Autodesk Fusion 360 part; units mm, degrees
sketch "Sketch1" plane through (0, 0, 0) normal (0, 0, 1) x (1, 0, 0)
  line L0 (55, 35) -> (117.913, 35)
  line L1 (117.913, 35) -> (117.913, -30.294)
  line L2 (117.913, -30.294) -> (55, -30.294)
  line L3 (55, -30.294) -> (55, 35)
  line L4 (44.5, -40.794) -> (127.413, -40.794)
  line L5 (127.413, -40.794) -> (127.413, 44.5)
  line L6 (127.413, 44.5) -> (44.5, 44.5)
  line L7 (44.5, 44.5) -> (44.5, -40.794)
  circle A0 centre (49.5, -35.794) radius 1.7
  circle A1 centre (49.5, 39.5) radius 1.7
  circle A2 centre (122.413, 39.5) radius 1.7
  circle A3 centre (122.413, -35.794) radius 1.7
  circle A4 centre (49.5, -35.794) radius 3
  circle A5 centre (49.5, 39.5) radius 3
  circle A6 centre (122.413, 39.5) radius 3
  circle A7 centre (122.413, -35.794) radius 3
  dimension "d1" = 62.913
  dimension "d2" = 65.294
  dimension "d3" = 82.913
  dimension "d4" = 85.294
  dimension "d5" = 9.5
  dimension "d6" = 9.5
  dimension "d7" = 3.4
  dimension "d8" = 3.4
  dimension "d9" = 3.4
  dimension "d10" = 3.4
  dimension "d11" = 5
  dimension "d12" = 5
  dimension "d13" = 5
  dimension "d14" = 5
  dimension "d15" = 5
  dimension "d16" = 5
  dimension "d17" = 5
  dimension "d18" = 5
  dimension "d19" = 6
  dimension "d20" = 6
  dimension "d21" = 6
  dimension "d22" = 6
extrude "Extrude1" add sketch "Sketch1" along normal blind 9.9 from surface at 3.1 contours A4 | A5 | A6 | A7 makes body 1 at (123.2255, -32.9061, 9.7) makes body 2 at (123.2255, 42.3879, 9.7) makes body 3 at (46.5037, -35.9435, 9.7) makes body 4 at (46.5037, 39.3505, 9.7)
extrude "Extrude2" add sketch "Sketch1" along normal blind 13 contours L4 L5 L6 L7 bodies 1 2 3 4
extrude "Extrude3" add sketch "Sketch1" along normal blind 3 contours L0 L1 L2 L3 bodies 1
sketch "Sketch2" plane through (0, 0, 13) normal (0, 0, 1) x (-1, 0, 0)
  circle A0 centre (-122.413, 35.794) radius 1.7
  circle A1 centre (-49.5, -39.5) radius 1.7
  line L0 (-117.913, 30.294) -> (-55, 30.294)
  line L1 (-55, 30.294) -> (-55, -35)
  line L2 (-55, -35) -> (-117.913, -35)
  line L3 (-117.913, -35) -> (-117.913, 30.294)
  line L4 (-44.5, -44.5) -> (-44.5, 40.794)
  line L5 (-44.5, 40.794) -> (-127.413, 40.794)
  line L6 (-127.413, 40.794) -> (-127.413, -44.5)
  line L7 (-127.413, -44.5) -> (-44.5, -44.5)
  circle A2 centre (-122.413, -39.5) radius 1.7
  circle A3 centre (-49.5, 35.794) radius 1.7
  line L8 (-76.7065, -44.5) -> (-95.2065, -44.5)
  line L9 (-95.2065, -44.5) -> (-95.2065, -35)
  line L10 (-95.2065, -35) -> (-76.7065, -35)
  line L11 (-76.7065, -35) -> (-76.7065, -44.5)
  line L12 (-44.5, -44.5) -> (-44.5, 40.794)
  dimension "d30" = 18.5
  dimension "d31" = 32.2065
extrude "Extrude4" cut sketch "Sketch2" against normal blind 7.5 contours L2 L7 L8 L9 L10 L11 bodies 1
fillet "Fillet1" radius 5 4 edges at (44.5, 44.5, 6.5) (44.5, -40.794, 6.5) (127.413, 44.5, 6.5) (127.413, -40.794, 6.5) on bodies 1
sketch "Sketch3" plane through (0, 0, 13) normal (0, 0, 1) x (-1, 0, 0)
  circle A0 centre (-49.5, 35.794) radius 1.7
  circle A1 centre (-122.413, -39.5) radius 1.7
  arc A2 (-122.413, 40.794) -> (-127.413, 35.794) centre (-122.413, 35.794) ccw
  line L0 (-127.413, 35.794) -> (-127.413, -39.5)
  arc A3 (-127.413, -39.5) -> (-122.413, -44.5) centre (-122.413, -39.5) ccw
  line L1 (-122.413, -44.5) -> (-95.2065, -44.5)
  line L2 (-95.2065, -44.5) -> (-95.2065, -35)
  line L3 (-95.2065, -35) -> (-117.913, -35)
  line L4 (-117.913, -35) -> (-117.913, 30.294)
  line L5 (-117.913, 30.294) -> (-55, 30.294)
  line L6 (-55, 30.294) -> (-55, -35)
  line L7 (-55, -35) -> (-76.7065, -35)
  line L8 (-76.7065, -35) -> (-76.7065, -44.5)
  line L9 (-76.7065, -44.5) -> (-49.5, -44.5)
  arc A4 (-49.5, -44.5) -> (-44.5, -39.5) centre (-49.5, -39.5) ccw
  line L10 (-44.5, -39.5) -> (-44.5, 35.794)
  arc A5 (-44.5, 35.794) -> (-49.5, 40.794) centre (-49.5, 35.794) ccw
  line L11 (-49.5, 40.794) -> (-122.413, 40.794)
  circle A6 centre (-49.5, -39.5) radius 1.7
  circle A7 centre (-122.413, 35.794) radius 1.7
sketch "Sketch4" plane through (0, 0, 13) normal (0, 0, 1) x (-1, 0, 0)
The listing builds one solid part. Answer for the finished solid, in the listing's coordinates (mm). A direction names the side the tool comes from. Round coordinates to 2 decimals unless told otherwise and drop trailing zeros. Order: outer loops, then holes, each group sorted by start corner. A loop starts at its lowest first (then second) coordinate and runs counter-clockwise, first axis right, second up. Notation, with made-up numbers: (74, 64.5) - (102, 64.5) arc R9 ccw to (102, 80.5) - close; hole circle Ø10 at (-34, 80.5). An arc over 180 degrees is marked (long way). Write item = value, one per line. Start each with the question number.
1) For a pull along X with two mould halves and no side action, classify faces 5 (the cylindrical face through (121.06, 40.53, 7.98)), 6 (the cylindrical face through (47.29, 37.47, 1.53)), 7 (the flat face through (44.5, 2, 6)), 8 (the flat face through (85, -40.794, 6)) as released by +X, released by -X, zero draft, split by the parting line, or undercut.
2) For faces 1 (the cylindrical face through (125.987, 42.996, 6.591)), 2 (the flat face through (86, 3, 3)), 3 (the flat face through (76.706, 40, 9)), 4 (the cylindrical face through (125.274, 38.599, 1.528)), determine the directions among +Z, -Z, +X, -X, +Y, -Y from which every point of the face is accessible in a straight line to the end or side of a thin tool.
3) Section B-B, the plane x = 79 is taken. Write down the section's boundary in (y, z).
4) Section C-C, the plane y = -26.5 is taken. Write down the section's boundary in (x, z), plus the area to 3 significant figures.
5) Section A-A, the plane z = 7.75 is taken. Write down the section's boundary in (x, y), plus the area to 3 significant figures.
6) Given pin 1 (4 mm diameter, centred on x = 61, y = 15, fed in from +Z); pin 2 (1.8 mm diameter, centred on x = 50.5, y = -35.5, fed in from -Z); pin 3 (5 mm diameter, centred on x = 90, y = 42, fed in from +Z), each flat-ended and moving along its own axis, determine where each tip first touches the part or whether it passes through.
7) Straight lines are drawn through the part: L1, parallel to Y at x = 49.5, z = 2.3; L2, parallel to Y at x = 49.5, z = 11; L3, parallel to Y at x = 116, z = 4.75. For each, find the intervals that lie inside material, in ascending order.
Results list:
q1.face_5 = undercut
q1.face_6 = undercut
q1.face_7 = released by -X
q1.face_8 = zero draft
q2.face_1 = +Z, -Z, +X, +Y
q2.face_2 = +Z
q2.face_3 = +Z, +Y
q2.face_4 = -Z
q3.outline = (-40.79, 0) - (44.5, 0) - (44.5, 5.5) - (35, 5.5) - (35, 3) - (-30.29, 3) - (-30.29, 13) - (-40.79, 13) - close
q4.outline = (44.5, 0) - (127.41, 0) - (127.41, 13) - (117.91, 13) - (117.91, 3) - (55, 3) - (55, 13) - (44.5, 13) - close
q4.area = 449 mm^2
q5.outline = (44.5, -35.79) arc R5 ccw to (49.5, -40.79) - (122.41, -40.79) arc R5 ccw to (127.41, -35.79) - (127.41, 39.5) arc R5 ccw to (122.41, 44.5) - (95.21, 44.5) - (95.21, 35) - (117.91, 35) - (117.91, -30.29) - (55, -30.29) - (55, 35) - (76.71, 35) - (76.71, 44.5) - (49.5, 44.5) arc R5 ccw to (44.5, 39.5) - close; hole circle Ø3.4 at (49.5, -35.79); hole circle Ø3.4 at (49.5, 39.5); hole circle Ø3.4 at (122.41, -35.79); hole circle Ø3.4 at (122.41, 39.5)
q5.area = 2,730 mm^2
q6.pin_1 = 3
q6.pin_2 = 3.1
q6.pin_3 = 5.5
q7.L1 = -40.79 to -38.79, -32.79 to 36.5, 42.5 to 44.5
q7.L2 = -40.79 to -37.49, -34.09 to 37.8, 41.2 to 44.5
q7.L3 = -40.79 to -30.29, 35 to 44.5
